```python
from build123d import *

# Parameters (mm, degrees)
F1_DEPTH = 11.5
F3_DEPTH = 10.5
F4_W     = 57.923077
F4_H     = 25.561713
F5_DEPTH = 7.5
F6_W     = 35
F6_H     = 5.974728
F7_DEPTH = 5


with BuildPart() as f1:
    # F0 (on Top) → F1 (new body, symmetric)
    with BuildSketch(Plane.XY):
        Polygon((52.666136, 19.229225), (-48.333864, 19.229225), (-54.333864, -5.270775), (52.666136, -5.270775), align=None)
    extrude(amount=F1_DEPTH, both=True)

    # F2 (on Top) → F3 (cut, symmetric)
    with BuildSketch(Plane.XY):
        Polygon((13.666136, -4.270775), (53.666136, -4.270775), (53.666136, 16.229225), (-47.907322, 16.229225), (-53.662424, -7.270775), (13.666136, -7.270775), align=None)
    extrude(amount=F3_DEPTH, both=True, mode=Mode.SUBTRACT)

    # F4 (on Top) → F5 (cut, symmetric)
    with BuildSketch(Plane.XY):
        with Locations((33.046458, -3.861708)):
            Rectangle(F4_W, F4_H)
    extrude(amount=F5_DEPTH, both=True, mode=Mode.SUBTRACT)

    # F6 (on Top) → F7 (cut, symmetric)
    with BuildSketch(Plane.XY):
        with Locations((-2.833864, 15.241861)):
            Rectangle(F6_W, F6_H)
    extrude(amount=F7_DEPTH, both=True, mode=Mode.SUBTRACT)


solid = f1.part
```
Input: part model. Units: mm. Frame: model coordinates. A direction names the side the tool comes from. Give positions to 0.01 mm unless a question says otherwise; leave off trailing zeros. Order: outer loops, then holes, each group sorted by start corner. A loop starts at its lowest first (then second) coordinate and runs counter-clockwise, first axis right, second up. Notation, with made-up numbers: (4.5, 12) - (12.5, 12) arc R26 ccw to (12.5, 29) - close; hole circle Ø3 at (8, 37). An arc over 180 degrees is marked (long way). One line per item, written item: value.
1. Draft query along Y for faces 4 (the face through (-51.29, 7.15, 0.16)), 5 (the face through (52.666, 17, 1)), 6 (the face through (3, 16.229, 7)), 7 (the face through (33, -4.271, -9)). Return one class per face: released by +Y, released by -Y, zero draft, split by the parting line, or undercut.
Determined:
face 4: released by +Y
face 5: zero draft
face 6: undercut
face 7: undercut
2. Cut plane D-D, the plane y = -1.75. Output: boundary loops of the cut face in (x, z).
Determined:
outline: (-53.47, -11.5) - (52.67, -11.5) - (52.67, -10.5) - (-52.31, -10.5) - (-52.31, 10.5) - (52.67, 10.5) - (52.67, 11.5) - (-53.47, 11.5) - close
3. Cut plane B-B, the plane x = -30. Output: boundary loops of the cut face in (y, z), and give its area (3 significant figures).
Determined:
outline: (-5.27, -11.5) - (19.23, -11.5) - (19.23, 11.5) - (-5.27, 11.5) - (-5.27, 10.5) - (16.23, 10.5) - (16.23, -10.5) - (-5.27, -10.5) - close
area: 112 mm2
4. Cut plane C-C, the plane z = 0. Output: boundary loops of the cut face in (x, y).
Determined:
outline: (-54.33, -5.27) - (-53.17, -5.27) - (-47.91, 16.23) - (-20.33, 16.23) - (-20.33, 18.23) - (14.67, 18.23) - (14.67, 16.23) - (52.67, 16.23) - (52.67, 19.23) - (-48.33, 19.23) - close
5. Cut plane A-A, the plane z = -9.5. Output: boundary loops of the cut face in (x, y), and give its area (3 significant figures).
Determined:
outline: (-54.33, -5.27) - (-53.17, -5.27) - (-47.91, 16.23) - (52.67, 16.23) - (52.67, 19.23) - (-48.33, 19.23) - close; (13.67, -5.27) - (52.67, -5.27) - (52.67, -4.27) - (13.67, -4.27) - close
area: 368 mm2
6. Reachability of faces 1 (the face through (-20.334, 17, 0)), 2 (the face through (-2, 7, -11.5)), 3 (the face through (33, -4.271, 9)) from +Z, -Z, +X, -X, +Y, -Y: full face, straight path, thin tool, end or side. Return the list, or none.
Determined:
face 1: -Y
face 2: -Z, +X, -X, +Y, -Y
face 3: +X
7. Pin query (flat end, axial travel): pin 1 Ø12 at (x, z) = (-22, 1.5) entering from -Y; pin 2 Ø1.1 at (y, z) = (-5, -9.5) entering from -X; pin 3 Ø1.6 at (y, z) = (17.5, 0) entering from -X; pin 4 Ø5 at (y, z) = (5, -3.5) entering from +X. Return the tip coordinate at first contact, or that it passes through.
Determined:
pin 1: y = 16.23
pin 2: x = -54.33
pin 3: x = -48.95
pin 4: x = -50.05
8. Line query: probe 1 along Z at (x, y) = (-10.5, 8.5); probe 2 along Y at (x, z) = (39, -9.75); probe 3 along Y at (x, z) = (-6, 2.5). Output: solid intervals per line, ascending.
Determined:
probe 1: -11.5 to -10.5, 10.5 to 11.5
probe 2: -5.27 to -4.27, 16.23 to 19.23
probe 3: 18.23 to 19.23
